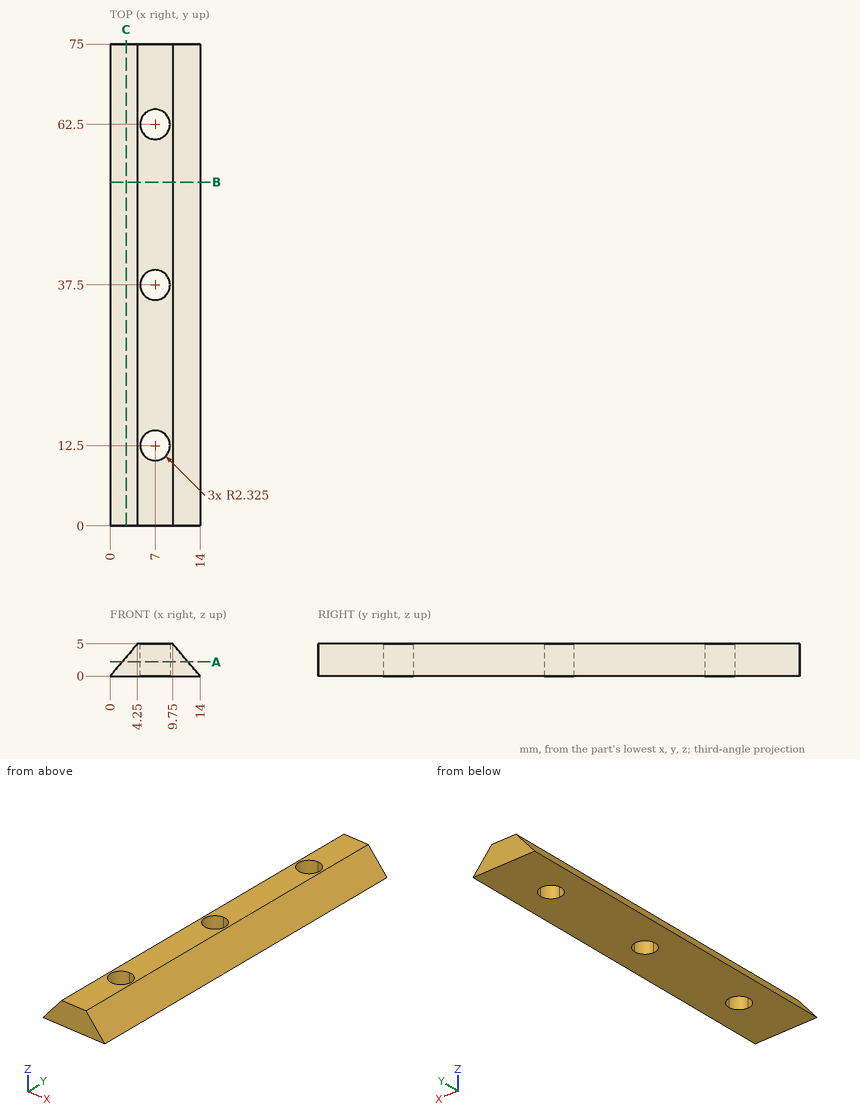
The drawing under review shows one solid part. Ordinate dimensions are in mm from its lowest x, y, z. Give positions to 0.01 mm unless a question says otherwise; leave off trailing zeros. Write each loop counter-clockwise with the first axis right and the second up, starting at its lowest first coordinate (ties: lowest second). Pieces come first, ordered by that corner, then holes. Notation, with made-up numbers: (21.25, 77) -> (33.25, 77) arc R19 cw to (33.25, 107) -> close; hole circle Ø1 at (85.5, 41.25). An arc over 180 degrees is marked (long way). Answer in a Markdown table with one row per item.
(1) To check wall thickness, follow probe 1 along Y at (x, z) = (5.5, 0.8); probe 2 along X at (y, z) = (14, 2.9) (3 decimals); probe 3 along Y at (x, z) = (6, 4.45). State the ranges of each line that lie inside material, in increasing order.
Results:
| item | result |
|---|---|
| probe 1 | 0 to 10.72, 14.28 to 35.72, 39.28 to 60.72, 64.28 to 75 |
| probe 2 | 2.465 to 5.224, 8.776 to 11.535 |
| probe 3 | 0 to 10.4, 14.6 to 35.4, 39.6 to 60.4, 64.6 to 75 |
(2) Consider section C-C (x = 2.5). State the section outline as (y, z) points.
Results:
| item | result |
|---|---|
| outline | (0, 0) -> (75, 0) -> (75, 2.94) -> (0, 2.94) -> close |
(3) Consider section B-B (y = 53.5). State the section outline as (x, z) points, then the cut area to 4 significant figures.
Results:
| item | result |
|---|---|
| outline | (0, 0) -> (14, 0) -> (9.75, 5) -> (4.25, 5) -> close |
| area | 48.75 mm2 |
(4) Clearance check with a flat-ended pin moving along its axis: pin 1 (2 mm diameter, centred on y = 61.5, z = 3, fed in from +X). State where the tip first meets the part, or that it passes through.
Results:
| item | result |
|---|---|
| pin 1 | x = 12.3 |
(5) Consider section A-A (z = 2.2). State the section outline as (x, y) points (3 decimals).
Results:
| item | result |
|---|---|
| outline | (1.87, 0) -> (12.13, 0) -> (12.13, 75) -> (1.87, 75) -> close; hole (7, 14.825) arc R2.325 ccw (long way) to (9.325, 12.5) arc R2.325 ccw to start; hole (7, 39.825) arc R2.325 ccw (long way) to (9.325, 37.5) arc R2.325 ccw to start; hole (7, 64.825) arc R2.325 ccw (long way) to (9.325, 62.5) arc R2.325 ccw to start |
